```python
from build123d import *

# Parameters (mm, degrees)
PAD009_DEPTH        = 920
SKETCH017_W         = 220
SKETCH017_H         = 55
SKETCH017_W_2       = 320
SKETCH017_H_2       = 5
POCKET002_DEPTH     = 20
LINEARPATTERN_COUNT = 9
LINEARPATTERN_PITCH = 100


with BuildPart() as part:
    # Sketch016 → Pad009 (new body)
    with BuildSketch(Plane.XY):
        with BuildLine():
            Line((20, 0), (305, 0))
            ThreePointArc((305, 0), (319.142136, 5.857864), (325, 20))
            Line((325, 20), (325, 435))
            Line((325, 435), (0, 435))
            Line((0, 435), (0, 20))
            ThreePointArc((0, 20), (5.857864, 5.857864), (20, 0))
        make_face()
    extrude(amount=PAD009_DEPTH)

    # Sketch017 → Pocket002 (cut)
    with BuildSketch(Plane.XZ):
        with Locations((160, 47.5)):
            Rectangle(SKETCH017_W, SKETCH017_H)
        with Locations((160, 97.5)):
            Rectangle(SKETCH017_W_2, SKETCH017_H_2)
    pocket002 = extrude(amount=-POCKET002_DEPTH, mode=Mode.SUBTRACT)

    # LinearPattern: Pocket002 ×9
    with Locations(*[(0, 0, i * LINEARPATTERN_PITCH) for i in range(1, LINEARPATTERN_COUNT)]):
        add(pocket002, mode=Mode.SUBTRACT)


solid = part.part
```
Can you work these out from the model? Positions are in its coordinate system, mm. A direction names the side the tool comes from. Give positions to 0.01 mm unless a question says otherwise; leave off trailing zeros. Loops run counter-clockwise (first coordinate to the right, second up) from the corner with the lowest first, then second, coordinate; pieces in that order, holes last. Notation, with made-up numbers: M 16.25,-21 L 33.25,-21 A17 cw 33.25,-6 Z; hole C 29,-30 d4. An arc over 180 degrees is marked long. Answer in a Markdown table with one row per item.
1. Which directions (+Z, -Z, +X, -X, +Y, -Y) give clear straight access to the entire face, cutting with the end or side of a thin tool? Please do faces 1 (the cylindrical face through (318.986, 5.703, 453.56)), 2 (the flat face through (270, 10, 747)), 3 (the flat face through (158, 10, 795)).
Taken from the geometry:
| item | result |
|---|---|
| face 1 | +Z, -Z, +X, -Y |
| face 2 | -Y |
| face 3 | -X, -Y |
2. Suppose I cut it at A-A on z = 535. Write out the boundary of the cut face in (x, y).
Taken from the geometry:
| item | result |
|---|---|
| outline | M 0,20 A20 ccw 20,0 L 50,0 L 50,20 L 270,20 L 270,0 L 305,0 A20 ccw 325,20 L 325,435 L 0,435 Z |
3. For pin 1 Ø1 at (x, z) = (202.5, 444.5) entering from -Y; pin 2 Ø6 at (x, y) = (94.5, 13.5) entering from -Z; pin 3 Ø6 at (y, z) = (11, 356.5) entering from +X; pin 4 Ø6 at (y, z) = (5.5, 642) entering from -X, each with a flat end and sliding along its axis, tell me the tip position at first contact or that it passes through.
Taken from the geometry:
| item | result |
|---|---|
| pin 1 | stops at y = 20 |
| pin 2 | stops at z = 0 |
| pin 3 | stops at x = 324.08 |
| pin 4 | stops at x = 3.64 |
4. If I drill on line 1 along Y through (x, z) = (142, 463); line 2 along Y through (x, z) = (309, 475), over which ranges is the centre line in solid material (lowest first)?
Taken from the geometry:
| item | result |
|---|---|
| line 1 | y = 20 to 435 |
| line 2 | y = 0.4 to 435 |
